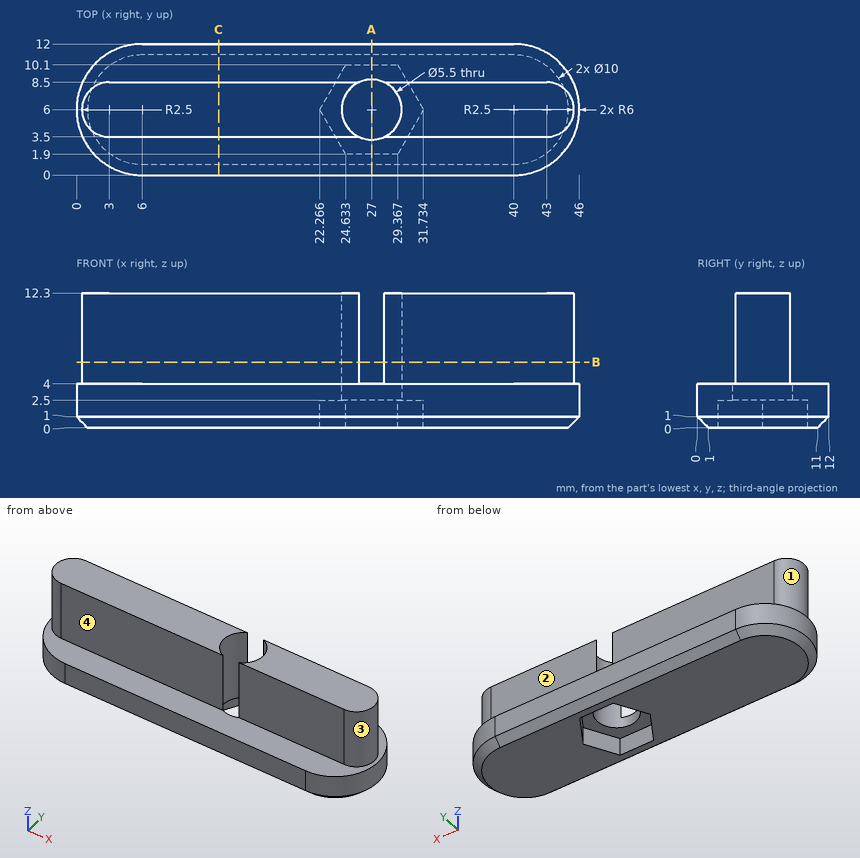
Part print with two shaded views. Sizes in mm from the minimum x, y, z corner. A direction names the side the tool comes from. Give positions to 0.01 mm unless a question says otherwise; leave off trailing zeros. Order: outer loops, then holes, each group sorted by start corner. A loop starts at its lowest first (then second) coordinate and runs counter-clockwise, first axis right, second up. Notation, with made-up numbers: M 76,-13.5 L 132,-13.5 A11 ccw 132,-5.5 Z; hole C 75.5,55 d6. An arc over 180 degrees is marked long. Put each result on its own line as item: value.
Item 1: Wall check: probe 1 along X at (y, z) = (6, 8.5); probe 2 along Z at (x, y) = (42, 3.25); probe 3 along X at (y, z) = (8.25, 10.5). Give the ranges that are in metal, low to high.
Results are:
probe 1: 0.5 to 24.25, 29.75 to 45.5
probe 2: 0 to 4
probe 3: 1.91 to 25.42, 28.58 to 44.09
Item 2: Cut at C-C on x = 13. Write the cut outline in (y, z), then the cut area to 3 significant figures.
Results are:
outline: M 0,1 L 1,0 L 11,0 L 12,1 L 12,4 L 8.5,4 L 8.5,12.3 L 3.5,12.3 L 3.5,4 L 0,4 Z
area: 88.5 mm2
Item 3: Cut at B-B on z = 6. Write the cut outline in (x, y), then the cut area to 3 significant figures.
Results are:
outline: M 3,3.5 L 25.85,3.5 A2.75 cw 25.85,8.5 L 3,8.5 A2.5 ccw Z; M 28.15,3.5 L 43,3.5 A2.5 ccw 43,8.5 L 28.15,8.5 A2.75 cw Z
area: 197 mm2
Item 4: Which spindle directions (+Z, -Z, +X, -X, +Y, -Y) get a long thin tool onto all of the face, cutting with end or side? Do the marked faces 1, 2, 3 and 4. Say none if no direction does.
Results are:
face 1: +Z, -X
face 2: +Z, +X, -X, +Y
face 3: +Z, +X
face 4: +Z, +X, -X, -Y
Item 5: Drop flat-ended pins along their axis: pin 1 Ø2.5 at (x, z) = (13.5, 9.5) entering from -Y; pin 2 Ø0.8 at (x, z) = (26.5, 1.5) entering from -Y; pin 3 Ø1.5 at (y, z) = (4, 7.5) entering from +X (1 decimal); pin 4 Ø4 at (x, z) = (18, 9.5) entering from +Y. Give the stop position or say it passes through.
Results are:
pin 1: y = 3.5
pin 2: y = 0
pin 3: x = 45.2
pin 4: y = 8.5
Item 6: Cut at A-A on x = 27. Write the cut outline in (y, z).
Results are:
outline: M 0,1 L 1,0 L 1.9,0 L 1.9,2.5 L 3.25,2.5 L 3.25,4 L 0,4 Z; M 8.75,2.5 L 10.1,2.5 L 10.1,0 L 11,0 L 12,1 L 12,4 L 8.75,4 Z
